```python
from build123d import *

# Parameters (mm, degrees)
EXTRUDE_1_DEPTH     = 3
CUT_EXTRUDE_1_REACH = 142.492
SKETCH_2_R          = 1.6
SKETCH_3_R          = 1.6
CUT_EXTRUDE_2_DEPTH = 3
SKETCH_4_R          = 2.1
CUT_EXTRUDE_3_DEPTH = 10
CUT_EXTRUDE_4_DEPTH = 10
SKETCH_6_W          = 90
SKETCH_6_H          = 5
CUT_EXTRUDE_5_DEPTH = 10
FILLET_1_R          = 2


with BuildPart() as part:
    # 草图1 → 凸台-拉伸1 (new body)
    with BuildSketch(Plane.XY):
        with BuildLine():
            Line((2, 0), (125, 0))
            ThreePointArc((125, 0), (126.414213562, 0.585786438), (127, 2))
            Line((127, 2), (127, 58))
            ThreePointArc((127, 58), (126.414213562, 59.414213562), (125, 60))
            Line((125, 60), (2, 60))
            ThreePointArc((2, 60), (0.585786438, 59.414213562), (0, 58))
            Line((0, 58), (0, 2))
            ThreePointArc((0, 2), (0.585786438, 0.585786438), (2, 0))
        make_face()
    extrude(amount=EXTRUDE_1_DEPTH)

    # 草图2 → 切除-拉伸1 (cut, up to next)
    with BuildSketch(Plane.XY.offset(3), mode=Mode.PRIVATE) as cut_extrude_1_sk1:
        with Locations((15, 3)):
            Circle(SKETCH_2_R)
    cut_extrude_1_tool1 = extrude(cut_extrude_1_sk1.sketch, amount=-CUT_EXTRUDE_1_REACH, mode=Mode.PRIVATE) & part.part
    # 草图2 → 切除-拉伸1 (cut, up to next)
    with BuildSketch(Plane.XY.offset(3), mode=Mode.PRIVATE) as cut_extrude_1_sk2:
        with Locations((40, 3)):
            Circle(SKETCH_2_R)
    cut_extrude_1_tool2 = extrude(cut_extrude_1_sk2.sketch, amount=-CUT_EXTRUDE_1_REACH, mode=Mode.PRIVATE) & part.part
    # 草图2 → 切除-拉伸1 (cut, up to next)
    with BuildSketch(Plane.XY.offset(3), mode=Mode.PRIVATE) as cut_extrude_1_sk3:
        with Locations((87, 3)):
            Circle(SKETCH_2_R)
    cut_extrude_1_tool3 = extrude(cut_extrude_1_sk3.sketch, amount=-CUT_EXTRUDE_1_REACH, mode=Mode.PRIVATE) & part.part
    # 草图2 → 切除-拉伸1 (cut, up to next)
    with BuildSketch(Plane.XY.offset(3), mode=Mode.PRIVATE) as cut_extrude_1_sk4:
        with Locations((112, 3)):
            Circle(SKETCH_2_R)
    cut_extrude_1_tool4 = extrude(cut_extrude_1_sk4.sketch, amount=-CUT_EXTRUDE_1_REACH, mode=Mode.PRIVATE) & part.part
    add(cut_extrude_1_tool1.solids().sort_by_distance((15, 3, 3))[0], mode=Mode.SUBTRACT)
    add(cut_extrude_1_tool2.solids().sort_by_distance((40, 3, 3))[0], mode=Mode.SUBTRACT)
    add(cut_extrude_1_tool3.solids().sort_by_distance((87, 3, 3))[0], mode=Mode.SUBTRACT)
    add(cut_extrude_1_tool4.solids().sort_by_distance((112, 3, 3))[0], mode=Mode.SUBTRACT)

    # 草图3 → 切除-拉伸2 (cut)
    with BuildSketch(Plane.XY.offset(3)):
        with Locations((3, 45)):
            Circle(SKETCH_3_R)
        with Locations((3, 25)):
            Circle(SKETCH_3_R)
        with Locations(Location((124, 25, 0), (0, 0, 180))):
            Circle(SKETCH_3_R)
        with Locations(Location((124, 45, 0), (0, 0, 180))):
            Circle(SKETCH_3_R)
    extrude(amount=-CUT_EXTRUDE_2_DEPTH, mode=Mode.SUBTRACT)

    # 草图4 → 切除-拉伸3 (cut)
    with BuildSketch(Plane.XY.offset(3)):
        with Locations((82, 35)):
            Circle(SKETCH_4_R)
        with Locations((34, 35)):
            Circle(SKETCH_4_R)
        with Locations((34, 25)):
            Circle(SKETCH_4_R)
        with Locations((82, 25)):
            Circle(SKETCH_4_R)
    extrude(amount=-CUT_EXTRUDE_3_DEPTH, mode=Mode.SUBTRACT)

    # 草图5 → 切除-拉伸4 (cut)
    with BuildSketch(Plane(origin=(0, 0, 0), x_dir=(-1, 0, 0), z_dir=(0, 0, -1))):
        with BuildLine():
            Line((-111, 50), (-111, 15))
            ThreePointArc((-111, 15), (-114, 12), (-117, 15))
            Line((-117, 15), (-117, 50))
            ThreePointArc((-117, 50), (-114, 53), (-111, 50))
        make_face()
        with BuildLine():
            Line((-100, 50), (-100, 15))
            ThreePointArc((-100, 15), (-103, 12), (-106, 15))
            Line((-106, 15), (-106, 50))
            ThreePointArc((-106, 50), (-103, 53), (-100, 50))
        make_face()
        with BuildLine():
            Line((-89, 50), (-89, 15))
            ThreePointArc((-89, 15), (-92, 12), (-95, 15))
            Line((-95, 15), (-95, 50))
            ThreePointArc((-95, 50), (-92, 53), (-89, 50))
        make_face()
        with BuildLine():
            Line((-67, 50), (-67, 15))
            ThreePointArc((-67, 15), (-70, 12), (-73, 15))
            Line((-73, 15), (-73, 50))
            ThreePointArc((-73, 50), (-70, 53), (-67, 50))
        make_face()
        with BuildLine():
            Line((-56, 50), (-56, 15))
            ThreePointArc((-56, 15), (-59, 12), (-62, 15))
            Line((-62, 15), (-62, 50))
            ThreePointArc((-62, 50), (-59, 53), (-56, 50))
        make_face()
        with BuildLine():
            Line((-45, 50), (-45, 15))
            ThreePointArc((-45, 15), (-48, 12), (-51, 15))
            Line((-51, 15), (-51, 50))
            ThreePointArc((-51, 50), (-48, 53), (-45, 50))
        make_face()
        with BuildLine():
            Line((-23, 50), (-23, 15))
            ThreePointArc((-23, 15), (-26, 12), (-29, 15))
            Line((-29, 15), (-29, 50))
            ThreePointArc((-29, 50), (-26, 53), (-23, 50))
        make_face()
        with BuildLine():
            Line((-12, 50), (-12, 15))
            ThreePointArc((-12, 15), (-15, 12), (-18, 15))
            Line((-18, 15), (-18, 50))
            ThreePointArc((-18, 50), (-15, 53), (-12, 50))
        make_face()
    extrude(amount=-CUT_EXTRUDE_4_DEPTH, mode=Mode.SUBTRACT)

    # 草图6 → 切除-拉伸5 (cut)
    with BuildSketch(Plane(origin=(0, 0, 0), x_dir=(-1, 0, 0), z_dir=(0, 0, -1))):
        with Locations((-65, 57.5)):
            Rectangle(SKETCH_6_W, SKETCH_6_H)
    extrude(amount=-CUT_EXTRUDE_5_DEPTH, mode=Mode.SUBTRACT)

    # 圆角1
    fillet_1_edges = [part.edges().sort_by_distance(p)[0] for p in [
        (110, 55, 1.5),
        (110, 60, 1.5),
        (20, 60, 1.5),
        (20, 55, 1.5),
    ]]
    fillet(fillet_1_edges, radius=FILLET_1_R)


solid = part.part
```
Model file for the job. Use its own axes, mm. A direction names the side the tool comes from. Coordinates: 2 decimals unless noted, no trailing zeros. Loops run counter-clockwise (first coordinate to the right, second up) from the corner with the lowest first, then second, coordinate; pieces in that order, holes last. Notation, with made-up numbers: (-34, -11.5) - (-5, -11.5) arc R20 cw to (-5, 11.5) - close; hole circle Ø6 at (7, -6). An arc over 180 degrees is marked (long way). Answer as a JSON object with one key per item and string values. Group by question number.
(1) Probe line 1 along Y through (x, z) = (82, 1.1); line 2 along Y through (x, z) = (124, 0.8); line 3 along Y through (x, z) = (13, 2.6). List the from-to ranges inside material, lowest first.
(2) Cut at A-A (x = 40). Give the cut face in (y, z), then the cut area to 3 significant figures.
(3) Cut at B-B (x = 82). Give the cut face in (y, z).
(4) Tool access for faces 4 (the face through (23, 33, 1)), 5 (the face through (66, 55, 1)): list every direction of +Z, -Z, +X, -X, +Y, -Y with a clear straight run to the whole face (end or side of a thin tool).
(5) Two-plate mould, pull along X, no slides. Class faces 1 (the face through (0, 30, 1)), 2 (the face through (26, 53, 1)), 3 (the face through (10, 60, 1)): released by +X, released by -X, zero draft, split by the parting line, or undercut.
(6) Cut at C-C (z = 1). State how many separate pieces and enclosed holes the cut face has, then the cut area to 3 significant figures.
(7) Flat gauge pin, fed straight in: pin 1 (1 mm diameter, centred on x = 84, z = 1.5, fed in from +Y). Where does the tip first touch, or does it go through?
Geometry says:
{
 "1": {"line 1": "y = 0 to 22.9, 27.1 to 32.9, 37.1 to 55", "line 2": "y = 0 to 23.4, 26.6 to 43.4, 46.6 to 60", "line 3": "y = 0 to 12.76, 52.24 to 60"},
 "2": {"outline": "(0, 0) - (1.4, 0) - (1.4, 3) - (0, 3) - close; (4.6, 0) - (55, 0) - (55, 3) - (4.6, 3) - close", "area": "155 mm^2"},
 "3": {"outline": "(0, 0) - (22.9, 0) - (22.9, 3) - (0, 3) - close; (27.1, 0) - (32.9, 0) - (32.9, 3) - (27.1, 3) - close; (37.1, 0) - (55, 0) - (55, 3) - (37.1, 3) - close"},
 "4": {"face 4": "+Z, -Z", "face 5": "+Z, -Z, +Y"},
 "5": {"face 1": "released by -X", "face 2": "undercut", "face 3": "zero draft"},
 "6": {"separate pieces": "1", "enclosed holes": "20", "area": "5,140 mm^2"},
 "7": {"pin 1": "stops at y = 55"}
}
